CAD build for the part. Positions are in the model's coordinates, mm. Coordinates: 2 decimals unless noted, no trailing zeros. Loops run counter-clockwise (first coordinate to the right, second up) from the corner with the lowest first, then second, coordinate; pieces in that order, holes last.
1) Saw through at C-C, the plane y = 487.5. Give the number of separate pieces and of enclosed holes in the cut face, and give its area (3 significant figures).
2) Pin check, flat tips, straight feed: pin 1 Ø1.5 at (y, z) = (505, 567.5) entering from +X; pin 2 Ø7 at (x, z) = (-167.5, 569.5) entering from -Y; pin 3 Ø10 at (x, z) = (36, 557) entering from -Y. Stop position of each tip, or through.
3) Wall check: line 1 along Z through (x, y) = (200.5, 663); line 2 along Y through (x, z) = (194.5, 557); line 3 along Y through (x, z) = (233, 573). Give the ranges that are in metal, low to high.
4) Saw through at A-A, the plane x = 82. Write the cut outline in (y, z), and give its area (3 significant figures).
```python
from build123d import *

# Parameters (mm, degrees)
BOSS_EXTRUDE1_DEPTH = 23.2
FILLET1_R           = 13.4
SHELL1_START        = 554.066138639
SHELL1_DEPTH        = 22.2
SHELL1_START_2      = -740.047251584
SHELL1_2_DEPTH      = 319.643616058
SHELL1_START_3      = 428.823224764
SHELL1_3_DEPTH      = 319.643616058
BOSS_EXTRUDE2_START = -0.6
BOSS_EXTRUDE2_DEPTH = 0.6


with BuildPart() as part:
    # Sketch1 → Boss-Extrude1 (new body)
    with BuildSketch(Plane(origin=(0, 0, 577.266138639), x_dir=(-1, 0, 0), z_dir=(0, 0, -1))):
        with BuildLine():
            Line((246.373543052, 767.588219351), (232.840577428, 767.588219351))
            Line((232.840577428, 767.588219351), (221.373543052, 767.588219351))
            Line((221.373543052, 767.588219351), (-342.073297304, 767.588219351))
            Line((-342.073297304, 767.588219351), (-353.54033168, 767.588219351))
            Line((-353.54033168, 767.588219351), (-367.073297304, 767.588219351))
            Line((-367.073297304, 767.588219351), (-389.449877126, 447.588219351))
            Line((-389.449877126, 447.588219351), (-375.949877126, 447.588219351))
            Line((-375.949877126, 447.588219351), (-364.449877126, 447.588219351))
            Line((-364.449877126, 447.588219351), (-311.549877126, 447.588219351))
            Line((-311.549877126, 447.588219351), (-311.549877126, 525.588219351))
            Line((-311.549877126, 525.588219351), (-311.490727804, 525.588219351))
            Line((-311.490727804, 525.588219351), (-239.490727804, 525.588219351))
            Line((-239.490727804, 525.588219351), (-224.106525446, 525.500426272))
            Line((-224.106525446, 525.500426272), (-224.106525446, 514.79475476))
            ThreePointArc((-224.106525446, 514.79475476), (-219.917813499, 523.880773359), (-210.625026727, 527.588219351))
            Line((-210.625026727, 527.588219351), (90.450122874, 527.588219351))
            ThreePointArc((90.450122874, 527.588219351), (99.259487157, 524.148297851), (103.406771195, 515.649004109))
            Line((103.406771195, 515.649004109), (103.406771195, 525.500426272))
            Line((103.406771195, 525.500426272), (103.450122874, 525.588219351))
            Line((103.450122874, 525.588219351), (190.850122874, 525.588219351))
            Line((190.850122874, 525.588219351), (190.850122874, 447.588219351))
            Line((190.850122874, 447.588219351), (243.750122874, 447.588219351))
            Line((243.750122874, 447.588219351), (255.21715725, 447.588219351))
            Line((255.21715725, 447.588219351), (255.250122874, 447.588219351))
            Line((255.250122874, 447.588219351), (268.750122874, 447.588219351))
            Line((268.750122874, 447.588219351), (246.373543052, 767.588219351))
        make_face()
    extrude(amount=BOSS_EXTRUDE1_DEPTH)

    # Fillet1
    fillet1_edges = [part.edges().sort_by_distance(p)[0] for p in [
        (378.261587215, 607.588219351, 577.266138639),
        (-257.561832963, 607.588219351, 577.266138639),
    ]]
    fillet(fillet1_edges, radius=FILLET1_R)

    # Shell1: read off the stored shape, not the designer's step
    # Shell1 outline → Shell1 (cut)
    with BuildSketch(Plane.XY.offset(SHELL1_START)):
        with BuildLine():
            Line((-245.441027966, 766.588219351), (-267.677754164, 448.588219351))
            Line((-267.677754164, 448.588219351), (-191.850122874, 448.588219351))
            Line((-191.850122874, 448.588219351), (-191.850122874, 526.588219351))
            Line((-191.850122874, 526.588219351), (-102.828644378, 526.588219351))
            Line((-102.828644378, 526.588219351), (-102.406771195, 525.73386847))
            Line((-102.406771195, 525.73386847), (-102.406771195, 521.870977135))
            ThreePointArc((-102.406771195, 521.870977135), (-97.307286684, 526.793927216), (-90.450122874, 528.588219351))
            Line((-90.450122874, 528.588219351), (210.625026727, 528.588219351))
            ThreePointArc((210.625026727, 528.588219351), (217.80980826, 526.683016464), (223.106525446, 521.468069601))
            Line((223.106525446, 521.468069601), (223.106525446, 526.494735851))
            Line((223.106525446, 526.494735851), (239.487874476, 526.588219351))
            Line((239.487874476, 526.588219351), (312.549877126, 526.588219351))
            Line((312.549877126, 526.588219351), (312.549877126, 448.588219351))
            Line((312.549877126, 448.588219351), (388.377508416, 448.588219351))
            Line((388.377508416, 448.588219351), (366.140782218, 766.588219351))
            Line((366.140782218, 766.588219351), (-245.441027966, 766.588219351))
        make_face()
    extrude(amount=SHELL1_DEPTH, mode=Mode.SUBTRACT)

    # Shell1 2 outline → Shell1 2 (add)
    with BuildSketch(Plane(origin=(0, 0, 0), x_dir=(0.9975640502598233, 0.06975647374413793, 0), z_dir=(0.06975647374413793, -0.9975640502598234, 0)).offset(SHELL1_START_2)):
        with BuildLine():
            ThreePointArc((406.32337267, 576.266138639), (415.091496757, 572.634262726), (418.72337267, 563.866138639))
            Line((418.72337267, 563.866138639), (418.72337267, 568.945508678))
            ThreePointArc((418.72337267, 568.945508678), (415.798603538, 573.341369507), (411.40274271, 576.266138639))
            Line((411.40274271, 576.266138639), (406.32337267, 576.266138639))
        make_face()
    extrude(amount=SHELL1_2_DEPTH)

    # Shell1 3 outline → Shell1 3 (add)
    with BuildSketch(Plane(origin=(0, 0, 0), x_dir=(0.9975640502598233, -0.06975647374413843, 0), z_dir=(0.06975647374413843, 0.9975640502598233, 0)).offset(SHELL1_START_3)):
        with BuildLine():
            ThreePointArc((-285.917636954, -576.266138639), (-294.68576104, -572.634262725), (-298.317636954, -563.866138639))
            Line((-298.317636954, -563.866138639), (-298.317636953, -568.94550868))
            ThreePointArc((-298.317636953, -568.94550868), (-295.392867822, -573.341369507), (-290.997006994, -576.266138639))
            Line((-290.997006994, -576.266138639), (-285.917636954, -576.266138639))
        make_face()
    extrude(amount=SHELL1_3_DEPTH)

    # Sketch2 → Boss-Extrude2 (add)
    with BuildSketch(Plane(origin=(0, 0, 554.066138639), x_dir=(-1, 0, 0), z_dir=(0, 0, -1)).offset(BOSS_EXTRUDE2_START)):
        with BuildLine():
            Line((246.373543052, 767.588219351), (-367.073297304, 767.588219351))
            Line((-367.073297304, 767.588219351), (-389.449877126, 447.588219351))
            Line((-389.449877126, 447.588219351), (-311.549877126, 447.588219351))
            Line((-311.549877126, 447.588219351), (-311.549877126, 525.588219351))
            Line((-311.549877126, 525.588219351), (-311.312198799, 525.588219351))
            Line((-311.312198799, 525.588219351), (-239.490727804, 525.588219351))
            Line((-239.490727804, 525.588219351), (-224.106525446, 525.500426272))
            Line((-224.106525446, 525.500426272), (-224.106525446, 514.79475476))
            ThreePointArc((-224.106525446, 514.79475476), (-219.917813499, 523.880773359), (-210.625026727, 527.588219351))
            Line((-210.625026727, 527.588219351), (90.450122874, 527.588219351))
            ThreePointArc((90.450122874, 527.588219351), (99.259487157, 524.148297851), (103.406771195, 515.649004109))
            Line((103.406771195, 515.649004109), (103.406771195, 525.500426272))
            Line((103.406771195, 525.500426272), (103.450122874, 525.588219351))
            Line((103.450122874, 525.588219351), (190.612444548, 525.588219351))
            Line((190.612444548, 525.588219351), (190.850122874, 525.588219351))
            Line((190.850122874, 525.588219351), (190.850122874, 525.176548414))
            Line((190.850122874, 525.176548414), (190.850122874, 447.588219351))
            Line((190.850122874, 447.588219351), (268.750122874, 447.588219351))
            Line((268.750122874, 447.588219351), (246.373543052, 767.588219351))
        make_face()
    extrude(amount=BOSS_EXTRUDE2_DEPTH)


solid = part.part
```
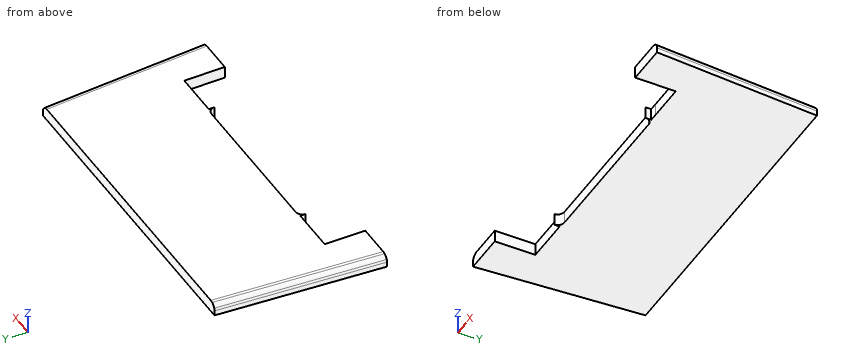
Data:
1. separate pieces: 2
1. enclosed holes: 2
1. area: 316 mm2
2. pin 1: stops at x = 385.13
2. pin 2: stops at y = 525.59
2. pin 3: stops at y = 527.59
3. line 1: z = 554.07 to 554.67, 576.27 to 577.27
3. line 2: y = 527.59 to 528.59, 766.59 to 767.59
3. line 3: y = 525.55 to 526.55, 766.59 to 767.59
4. outline: (527.59, 554.07) - (767.59, 554.07) - (767.59, 577.27) - (527.59, 577.27) - close; hole (528.59, 554.67) - (766.59, 554.67) - (766.59, 576.27) - (528.59, 576.27) - close
4. area: 427 mm2
